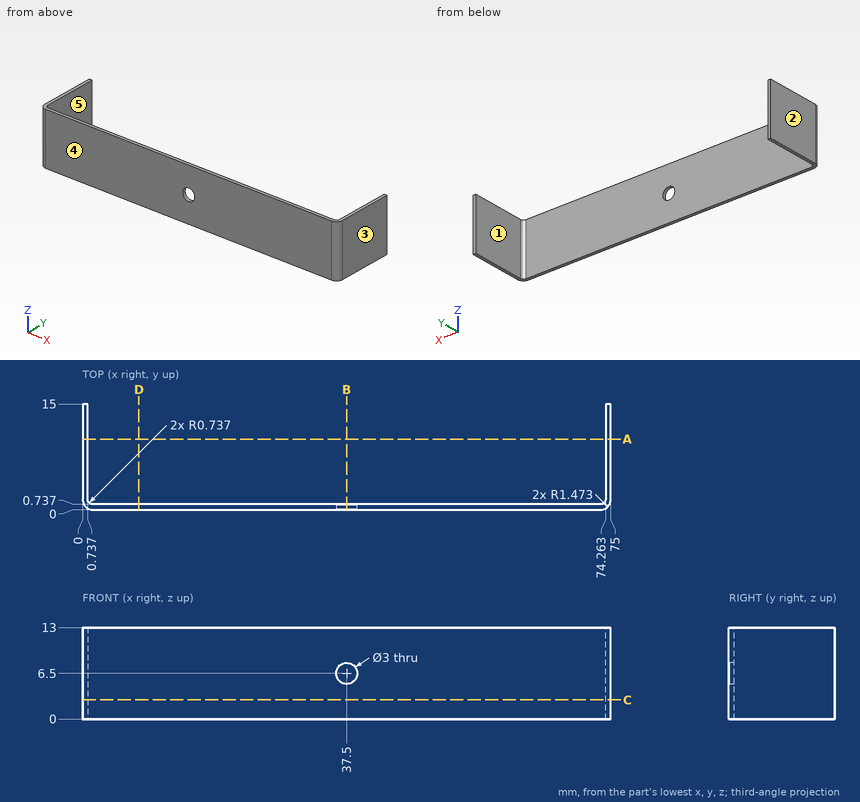
Here's the drawing with two shaded views (mm, measured from the low corner). I have some questions. A direction names the side the tool comes from. Coordinates: 2 decimals unless noted, no trailing zeros. Write each loop counter-clockwise with the first axis right and the second up, starting at its lowest first coordinate (ties: lowest second). Pieces come first, ordered by that corner, then holes. Notation, with made-up numbers: (28, 39) -> (53, 39) arc R26 cw to (53, 70) -> close; hole circle Ø11 at (63.5, 31). An arc over 180 degrees is marked (long way). One line per question, with ' | ' between items. Start each with the question number.
1. If we section it at D-D (x = 8): Please give me the cut outline in (y, z).
2. If we section it at C-C (z = 2.75): Please give me the cut outline in (x, y).
3. If we section it at A-A (y = 10): Please give me the cut outline in (x, z).
4. Thinking about a two-plate mould opening in X: for the marked faces 3, 4 and 5, which applies, pulls with the +X half, pulls with the -X half, needs draft (parallel to the pull), parting line crosses it, or undercut?
5. Will these pins go through, and if not, where does the flat tip stop? P1, Ø2.5, axis at x = 37.5, z = 6.5, coming from the -Y side; P2, Ø4, axis at x = 52, z = 5, coming from the +Y side.
6. If we section it at B-B (x = 37.5): Please give me the cut outline in (y, z).
7. For the marked faces 1 and 2, which set-ups out of +Z, -Z, +X, -X, +Y, -Y let a thin tool reach every point of the face, with its end or its side?
8. Please list where these lines run through material, in increasing order: line 1 along Z through (x, y) = (37.5, 0.45); line 2 along X through (y, z) = (6.75, 1.25); line 3 along X through (y, z) = (0.2, 6.5) (1 decimal).
Return value:
1) outline: (0, 0) -> (0.74, 0) -> (0.74, 13) -> (0, 13) -> close
2) outline: (0, 1.47) arc R1.47 ccw to (1.47, 0) -> (73.53, 0) arc R1.47 ccw to (75, 1.47) -> (75, 15) -> (74.26, 15) -> (74.26, 1.47) arc R0.74 cw to (73.53, 0.74) -> (1.47, 0.74) arc R0.74 cw to (0.74, 1.47) -> (0.74, 15) -> (0, 15) -> close
3) outline: (0, 0) -> (0.74, 0) -> (0.74, 13) -> (0, 13) -> close; (74.26, 0) -> (75, 0) -> (75, 13) -> (74.26, 13) -> close
4) face 3: pulls with the +X half | face 4: needs draft | face 5: undercut
5) P1: passes through | P2: stops at y = 0.74
6) outline: (0, 0) -> (0.74, 0) -> (0.74, 5) -> (0, 5) -> close; (0, 8) -> (0.74, 8) -> (0.74, 13) -> (0, 13) -> close
7) face 1: +Z, -Z, +Y | face 2: +Z, -Z, -X, +Y, -Y
8) line 1: z = 0 to 5, 8 to 13 | line 2: x = 0 to 0.74, 74.26 to 75 | line 3: x = 0.7 to 36, 39 to 74.3
